CAD build for the part. Positions are in the model's coordinates, mm. A direction names the side the tool comes from. Round coordinates to 2 decimals unless told otherwise and drop trailing zeros. Loops run counter-clockwise (first coordinate to the right, second up) from the corner with the lowest first, then second, coordinate; pieces in that order, holes last.
Autodesk Inventor part; units mm, degrees
ref_plane "YZ Plane" through (0, 0, 0) normal (1, 0, 0) x (0, 1, 0)
ref_plane "XZ Plane" through (0, 0, 0) normal (0, 1, 0) x (-1, 0, 0)
ref_plane "XY Plane" through (0, 0, 0) normal (0, 0, 1) x (1, 0, 0)
sketch "Sketch1" plane through (0, 0, 0) normal (0, 0, 1) x (1, 0, 0)
  line L0 (-9.6334, 0) -> (35.8666, 0)
  line L1 (35.8666, 0) -> (35.8666, 18.5)
  line L2 (35.8666, 18.5) -> (27.8666, 18.5)
  line L3 (27.8666, 18.5) -> (27.8666, 29.5)
  line L4 (27.8666, 29.5) -> (-3.4334, 29.5)
  line L5 (-3.4334, 29.5) -> (-3.4334, 15.3)
  line L6 (-3.4334, 15.3) -> (-9.6334, 15.3)
  line L7 (-9.6334, 0) -> (-9.6334, 15.3)
  point P0 (0, 0)
  dimension "d0" = 45.5
  dimension "d1" = 18.5
  dimension "d2" = 8
  dimension "d3" = 11
  dimension "d4" = 31.3
  dimension "d5" = 14.2
  dimension "d6" = 6.2
extrude "Extrusion1" add sketch "Sketch1" against normal blind 52
shell "Shell1" thickness 2 removed faces 1 at (7.5999, 5.1, 0)
sketch "Sketch2" plane through (-7.6334, 2, -50) normal (0, 0, 1) x (1, 0, 0)
  line L0 (41.5, 0) -> (0, 0)
  line L1 (0, 11.3) -> (6.2, 11.3)
  line L2 (6.2, 11.3) -> (6.2, 0)
  line L3 (6.2, 0) -> (0, 0)
  line L4 (0, 0) -> (0, 11.3)
  point P0 (7.6334, -2)
extrude "Extrusion2" add sketch "Sketch2" along normal blind 15.3
sketch "Sketch3" plane through (-1.4334, 2, -50) normal (0, 0, 1) x (1, 0, 0)
  line L0 (35.3, 0) -> (0, 0)
  line L1 (35.3, 14.5) -> (27.3, 14.5)
  line L2 (27.3, 14.5) -> (27.3, 0)
  line L3 (27.3, 0) -> (35.3, 0)
  line L4 (35.3, 0) -> (35.3, 14.5)
  point P0 (1.4334, -2)
extrude "Extrusion3" add sketch "Sketch3" along normal blind 7
sketch "Sketch4" plane through (0, 0, 0) normal (0, 0, 1) x (1, 0, 0)
  line L0 (-9.6334, 0) -> (35.8666, 0)
  line L1 (-7.6334, 2) -> (33.8666, 2)
  line L2 (33.8666, 2) -> (33.8666, 0)
  line L3 (33.8666, 0) -> (-7.6334, 0)
  line L4 (-7.6334, 0) -> (-7.6334, 2)
  point P0 (0, 0)
extrude "Extrusion4" cut sketch "Sketch4" against normal blind 151
sketch "Sketch5" plane through (-7.6334, 2, -52) normal (0, -1, 0) x (1, 0, 0)
  line L0 (41.5, 0) -> (0, 0)
  line L1 (41.5, 9) -> (41.5, 0)
  line L2 (41.5, 9) -> (33.5, 9)
  line L3 (33.5, 9) -> (33.5, 2)
  line L4 (33.5, 2) -> (6.2, 2)
  line L5 (6.2, 2) -> (6.2, 17.3)
  line L6 (6.2, 17.3) -> (0, 17.3)
  line L7 (0, 17.3) -> (0, 0)
  point P0 (7.6334, 52)
extrude "Extrusion5" add sketch "Sketch5" along normal blind 2
sketch "Sketch6" plane through (0, 0, 0) normal (0, 0, 1) x (1, 0, 0)
  line L0 (-3.4334, 29.5) -> (27.8666, 29.5)
  line L1 (27.8666, 29.5) -> (27.8666, 0)
  line L2 (27.8666, 0) -> (-3.4334, 0)
  line L3 (-3.4334, 0) -> (-3.4334, 29.5)
  line L4 (-9.6334, 15.3) -> (-3.4334, 15.3)
  line L5 (-3.4334, 15.3) -> (-3.4334, 0)
  line L6 (-3.4334, 0) -> (-9.6334, 0)
  line L7 (-9.6334, 0) -> (-9.6334, 15.3)
  line L8 (27.8666, 18.5) -> (35.8666, 18.5)
  line L9 (35.8666, 18.5) -> (35.8666, 0)
  line L10 (35.8666, 0) -> (27.8666, 0)
  line L11 (27.8666, 0) -> (27.8666, 18.5)
  point P0 (0, 0)
extrude "Extrusion6" add sketch "Sketch6" along normal blind 2
sketch "Sketch7" plane through (-9.6334, 0, -52) normal (-1, 0, 0) x (0, 0, 1)
  line L0 (0, 0) -> (0, 15.3)
  line L1 (54, 0) -> (0, 0)
  line L2 (21, 0) -> (33, 0)
  line L3 (33, 0) -> (33, 4.0069)
  line L4 (33, 4.0069) -> (21, 4.0069)
  line L5 (21, 4.0069) -> (21, 0)
  point P0 (52, 0)
  dimension "d20" = 54
  dimension "d21" = 12
  dimension "d22" = 21
extrude "Extrusion7" add sketch "Sketch7" along normal blind 2
sketch "Sketch8" plane through (-9.6334, 0, -52) normal (0, -1, 0) x (1, 0, 0)
  line L0 (45.5, 0) -> (45.5, 54)
  line L1 (45.5, 33) -> (47.5, 33)
  line L2 (47.5, 33) -> (47.5, 21)
  line L3 (47.5, 21) -> (45.5, 21)
  line L4 (45.5, 21) -> (45.5, 33)
  point P0 (9.6334, 52)
  dimension "d25" = 2
extrude "Extrusion8" add sketch "Sketch8" against normal blind 3
sketch "Sketch9" plane through (35.8666, 0, -19) normal (0, 0, 1) x (1, 0, 0)
  line L0 (2, 0) -> (0, 0)
  line L1 (2, 0) -> (2, 3)
  line L2 (0, 0) -> (0, 3)
  line L3 (0.454, 0) -> (2, 3)
  line L4 (2, 3) -> (2, 0)
  point P0 (-35.8666, 0)
extrude "Extrusion9" cut sketch "Sketch9" against normal blind 19.25
sketch "Sketch10" plane through (-9.6334, 0, -19) normal (0, 0, 1) x (1, 0, 0)
  line L0 (-2, 0) -> (-2, 4.0069)
  line L1 (0, 0) -> (-2, 0)
  line L2 (0, 0) -> (-0.454, 0)
  line L3 (-0.454, 0) -> (-2, 4.0069)
  line L4 (-2, 0) -> (-0.454, 0)
  line L5 (-2, 0) -> (-2, 4.0069)
  point P0 (9.6334, 0)
  dimension "d30" = 0.454
extrude "Extrusion10" cut sketch "Sketch10" against normal blind 34.5
sketch "Sketch11" plane through (0, 0, -52) normal (0, 0, -1) x (-1, 0, 0)
  circle A0 centre (-0.9313, 25.5293) radius 1.7905
  point P0 (0, 0)
extrude "Extrusion11" cut sketch "Sketch11" against normal blind 27.25
properties part number "SkateBox"
Item 1: Mould opens along X. For faces 5 (the flat face through (33.867, 8, -21)), 6 (the flat face through (-10.85, 1.98, -24.92)), 7 (the flat face through (-2, 0, -35)), 8 (the flat face through (27.867, 24, -25)) say: released by +X, released by -X, zero draft, split by the parting line, or undercut.
Verdict:
face 5: undercut
face 6: released by -X
face 7: zero draft
face 8: released by +X
Item 2: Wall check: L1, parallel to Z at x = 22, y = 6.25; L2, parallel to X at y = 11, z = -20; L3, parallel to X at y = 24, z = -21. Give the ranges that are in metal, low to high.
Verdict:
L1: z = -52 to -50, 0 to 2
L2: x = -9.63 to -7.63, 33.87 to 35.87
L3: x = -3.43 to -1.43, 25.87 to 27.87
Item 3: Cut at A-A (x = -7). List the corners of the cut face in (y, z).
Verdict:
outline: (0, -52) - (15.3, -52) - (15.3, 2) - (0, 2) - (0, 0) - (13.3, 0) - (13.3, -34.7) - (0, -34.7) - close
Item 4: Cut at D-D (x = 6). List the corners of the cut face in (y, z).
Verdict:
outline: (0, -52) - (29.5, -52) - (29.5, 2) - (0, 2) - (0, 0) - (27.5, 0) - (27.5, -50) - (0, -50) - close
Item 5: Cut at B-B (y = 12). List the corners of the cut face in (x, z).
Verdict:
outline: (-9.63, -52) - (35.87, -52) - (35.87, 2) - (-9.63, 2) - close; hole (-7.63, -34.7) - (-1.43, -34.7) - (-1.43, -50) - (25.87, -50) - (25.87, -43) - (33.87, -43) - (33.87, 0) - (-7.63, 0) - close
Item 6: 3-axis set-ups, long thin cutter, end or side, ignore diameter. For faces 1 (the flat face through (-11, 4.007, -25)), 2 (the flat face through (37, 2, -31)), 3 (the flat face through (37, 3, -25)), 4 (the flat face through (30, 16.5, -21)): which of +Z, -Z, +X, -X, +Y, -Y reach the whole face in a straight line?
Verdict:
face 1: +Z, -Z, -X, +Y
face 2: -Z, +X, +Y, -Y
face 3: +Z, -Z, +X, +Y
face 4: -Y
Item 7: Cut at C-C (z = -36.5). List the corners of the cut face in (x, y), plus the area to 3 significant figures.
Verdict:
outline: (-9.63, 0) - (-1.43, 0) - (-1.43, 27.5) - (25.87, 27.5) - (25.87, 16.5) - (33.87, 16.5) - (33.87, 0) - (35.87, 0) - (35.87, 18.5) - (27.87, 18.5) - (27.87, 29.5) - (-3.43, 29.5) - (-3.43, 15.3) - (-9.63, 15.3) - close
area: 283 mm2
Item 8: Flat gauge pins, fed straight in: P1, Ø6.5, axis at x = 32.5, z = -32.5, coming from the +Y side; P2, Ø3, axis at y = 9, z = -22.5, coming from the +X side; P3, Ø0.6, axis at x = 36.5, z = -27.5, coming from the +Y side; P4, Ø17, axis at y = 4.5, z = -24, coming from the -X side. Where does each tip first touch, or does it go through?
Verdict:
P1: stops at y = 18.5
P2: stops at x = 35.87
P3: stops at y = 3
P4: stops at x = -11.63
